from build123d import *

# Parameters (mm, degrees)
PAD001_DEPTH    = 3
SKETCH004_W     = 6
SKETCH004_H     = 8
POCKET002_DEPTH = 5
SKETCH005_R     = 1.7
HOLE_DEPTH      = 25
CHAMFER001_SIZE = 2
POCKET005_DEPTH = 5


with BuildPart() as part:
    # Sketch003 → Pad001 (new body)
    with BuildSketch(Plane.XY):
        Polygon((-30, 10), (30, 10), (30, -5), (15, -5), (15, -10), (-15, -10), (-15, -5), (-30, -5), align=None)
    extrude(amount=PAD001_DEPTH)

    # Sketch004 → Pocket002 (cut)
    with BuildSketch(Plane.XY):
        with Locations((0, 1)):
            Rectangle(SKETCH004_W, SKETCH004_H)
    extrude(amount=POCKET002_DEPTH, mode=Mode.SUBTRACT)

    # Sketch005 → Hole (cut)
    with BuildSketch(Plane.XY):
        with Locations((-15, 7.5)):
            Circle(SKETCH005_R)
        with Locations((15, 7.5)):
            Circle(SKETCH005_R)
        with Locations((-10, -7.5)):
            Circle(SKETCH005_R)
        with Locations((10, -7.5)):
            Circle(SKETCH005_R)
    extrude(amount=HOLE_DEPTH, mode=Mode.SUBTRACT)

    # Chamfer001
    chamfer001_edges = [part.edges().sort_by_distance(p)[0] for p in [
        (-30, 10, 1.5),
        (30, 10, 1.5),
        (-30, 2.5, 3),
        (-22.5, -5, 3),
        (-15, -7.5, 3),
        (15, -7.5, 3),
        (22.5, -5, 3),
        (30, 2.5, 3),
        (30, -5, 1.5),
        (15, -10, 1.5),
        (15, -5, 1.5),
        (-15, -10, 1.5),
        (-15, -5, 1.5),
        (-30, -5, 1.5),
    ]]
    chamfer(chamfer001_edges, length=CHAMFER001_SIZE)

    # Sketch014 → Pocket005 (cut)
    with BuildSketch(Plane.XY):
        with BuildLine():
            Line((-11.7, -7.5), (-11.7, -10))
            Line((-11.7, -10), (-8.3, -10))
            Line((-8.3, -10), (-8.3, -7.5))
            ThreePointArc((-8.3, -7.5), (-10, -5.8), (-11.7, -7.5))
        make_face()
        with BuildLine():
            Line((8.3, -7.5), (8.3, -10))
            Line((8.3, -10), (11.7, -10))
            Line((11.7, -10), (11.7, -7.5))
            ThreePointArc((11.7, -7.5), (10, -5.8), (8.3, -7.5))
        make_face()
    extrude(amount=POCKET005_DEPTH, mode=Mode.SUBTRACT)


solid = part.part
For this review, take the finished solid that the model builds, in its own axes (mm). A direction names the side the tool comes from. Round coordinates to 2 decimals unless told otherwise and drop trailing zeros. Order: outer loops, then holes, each group sorted by start corner. A loop starts at its lowest first (then second) coordinate and runs counter-clockwise, first axis right, second up. Notation, with made-up numbers: M 33.5,61.25 L 50.5,61.25 A10 ccw 50.5,78.25 Z; hole C 50.5,68 d1. An arc over 180 degrees is marked long. Write each question's results on one line, items separated by ' | '. Start each with the question number.
1. Add section A-A (y = -9). State the section outline as (x, z) points.
2. Add section D-D (x = -23). State the section outline as (y, z) points, then the cut area to 3 significant figures.
3. Clearance check with flat-ended pins moving along their axes: pin 1 Ø2.5 at (x, y) = (-15, 7.5) entering from -Z; pin 2 Ø1.1 at (x, z) = (22, 0.5) entering from -Y; pin 3 Ø1 at (y, z) = (-6, 1.5) entering from +X; pin 4 Ø0.8 at (y, z) = (-9, 1.5) entering from +X. State where each tip first meets the part, or that it passes through.
4. Tool access review of faces 5 (the face through (-3, 1, 1)), 6 (the face through (-15, -7.5, 0.5)), 7 (the face through (15, -7.5, 0.5)): name each direction out of +Z, -Z, +X, -X, +Y, -Y from which nothing blocks a thin tool from reaching the whole face with its end or side.
5. Add section C-C (z = 2.2). State how many separate pieces and enclosed holes the cut face has, then the cut area to 3 significant figures.
6. Add section B-B (y = 1). State the section outline as (x, z) points.
7. Draft analysis for pull direction X (two halves, no side actions). For faces 1 (the face through (23, -4, 2)), 2 (the face through (-8.3, -9, 1)), 3 (the face through (29, 9, 1)), 4 (the face through (-29, 9, 1)), state which applies: pulls with the +X half, pulls with the -X half, needs draft (parallel to the pull), parting line crosses it, or undercut.
8. To check wall thickness, follow L1, parallel to X at y = 7.5, z = 0.75; L2, parallel to Y at x = 2, z = 0.4; L3, parallel to X at y = 7.5, z = 2.05. State the ranges of each line that lie inside material, in increasing order. Write a range as [from, to].
Output values:
1) outline: M -14,0 L -11.7,0 L -11.7,3 L -13,3 L -14,2 Z; M -8.3,0 L 8.3,0 L 8.3,3 L -8.3,3 Z; M 11.7,0 L 14,0 L 14,2 L 13,3 L 11.7,3 Z
2) outline: M -5,0 L 10,0 L 10,3 L -3,3 L -5,1 Z | area: 43.0 mm^2
3) pin 1: through | pin 2: y = -5 | pin 3: x = 16.21 | pin 4: x = 14.4
4) face 5: +Z, -Z | face 6: +Z, -Z, -X, -Y | face 7: +Z, -Z, +X, -Y
5) separate pieces: 1 | enclosed holes: 3 | area: 882 mm^2
6) outline: M -30,0 L -3,0 L -3,3 L -28,3 L -30,1 Z; M 3,0 L 30,0 L 30,1 L 28,3 L 3,3 Z
7) face 1: needs draft | face 2: undercut | face 3: pulls with the +X half | face 4: pulls with the -X half
8) L1: [-30, -16.7], [-13.3, 13.3], [16.7, 30] | L2: [-10, -3], [5, 10] | L3: [-28.95, -16.7], [-13.3, 13.3], [16.7, 28.95]
